Check sheet for the modelled part. Datum: model origin and axes. Units: mm. Round coordinates to 2 decimals unless told otherwise and drop trailing zeros. Write each loop counter-clockwise with the first axis right and the second up, starting at its lowest first coordinate (ties: lowest second). Pieces come first, ordered by that corner, then holes.
from build123d import *

# Parameters (mm, degrees)
F0_W     = 124
F0_H     = 14
F1_DEPTH = 2
F2_R     = 4
F3_DEPTH = 25
F4_R     = 4
F5_DEPTH = 25
F6_R     = 6.99999


# Not quite as in the source:
# - a fillet or chamfer is up to 0.001 mm smaller than in the source, because OpenCascade refuses the exact size


with BuildPart() as f1:
    # F0 (on Front) → F1 (new body)
    with BuildSketch(Plane.XZ):
        Rectangle(F0_W, F0_H)
    extrude(amount=F1_DEPTH)

    # F2 (on face) → F3 (cut)
    with BuildSketch(Plane.XZ.offset(2)):
        with Locations((-55, 0)):
            Circle(F2_R)
    extrude(amount=-F3_DEPTH, mode=Mode.SUBTRACT)

    # F4 (on face) → F5 (cut)
    with BuildSketch(Plane.XZ.offset(2)):
        with Locations((55, 0)):
            Circle(F4_R)
    extrude(amount=-F5_DEPTH, mode=Mode.SUBTRACT)

    # F6 (radius 7 in the source; OpenCascade refuses exactly that, so slightly less here)
    f6_edges = [f1.edges().sort_by_distance(p)[0] for p in [
        (-62, -1, 7),
        (-62, -1, -7),
        (62, -1, 7),
        (62, -1, -7),
    ]]
    fillet(f6_edges, radius=F6_R)


solid = f1.part
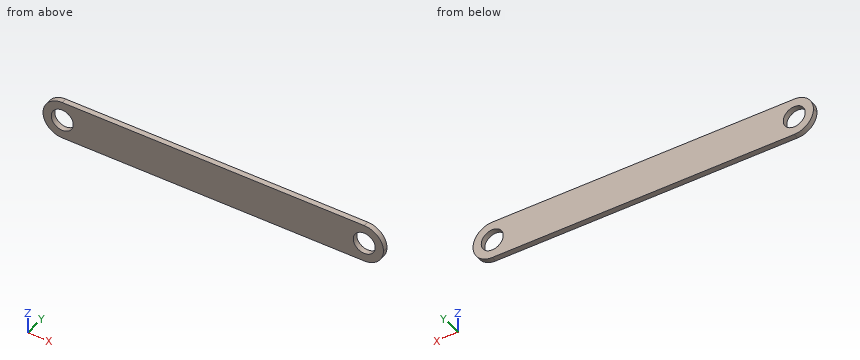
1. Sectioned sample at A-A, the plane y = -0.6. Give the number of separate pieces and of enclosed holes in the cut face, plus the area to 3 significant figures.
2. Scan lines: line 1 along Z through (x, y) = (55, -1.15); line 2 along X through (y, z) = (-1.4, -2.5); line 3 along Z through (x, y) = (53, -1.05). Record each from-to range of solid material in increasing order.
3. Sectioned sample at B-B, the plane z = -2.5. Enter the section's corners in (x, y), plus the area to 3 significant figures.
4. Go/stop test with a flat-tipped pin: pin 1 (6 mm diameter, centred on x = 4, z = 2, fed in from +Y). Record where the tip stops, or that it passes through.
Computed values:
1. separate pieces: 1
1. enclosed holes: 2
1. area: 1,590 mm2
2. line 1: z = -7 to -4, 4 to 7
2. line 2: x = -61.54 to -58.12, -51.88 to 51.88, 58.12 to 61.54
2. line 3: z = -7 to -3.46, 3.46 to 7
3. outline: (-61.54, -2) - (-58.12, -2) - (-58.12, 0) - (-61.54, 0) - close; (-51.88, -2) - (51.88, -2) - (51.88, 0) - (-51.88, 0) - close; (58.12, -2) - (61.54, -2) - (61.54, 0) - (58.12, 0) - close
3. area: 221 mm2
4. pin 1: stops at y = 0
